Part model, mm, in its own coordinate system. A direction names the side the tool comes from. Round coordinates to 2 decimals unless told otherwise and drop trailing zeros. Order: outer loops, then holes, each group sorted by start corner. A loop starts at its lowest first (then second) coordinate and runs counter-clockwise, first axis right, second up. Notation, with made-up numbers: (-20.5, 17.5) - (34.5, 17.5) arc R26 cw to (34.5, 51.5) - close; hole circle Ø5 at (87.5, -20). An arc over 180 degrees is marked (long way). Return JSON: item names as keys, results as strings. Group by question number.
Item 1: Drop flat-ended pins along their axis: pin 1 (10 mm diameter, centred on x = -17, z = 13, fed in from +Y); pin 2 (14.5 mm diameter, centred on x = 13, y = -3.5, fed in from +Z); pin 3 (7.5 mm diameter, centred on y = -1.5, z = 18, fed in from -X); pin 4 (1 mm diameter, centred on x = 2.5, y = 1, fed in from -Z). Give the stop position or say it passes through.
Item 2: Two-plate mould, pull along X, no slides. Class faces 1 (the face through (-14, 4.826, 20)), 2 (the face through (-0.252, 21.445, 7.776)), 3 (the face through (8, 0, 15.773)): released by +X, released by -X, zero draft, split by the parting line, or undercut.
Item 3: Probe probe 1 along X at (y, z) = (-4.5, 9.5); probe 2 along X at (y, z) = (4, 8); probe 3 along Z at (x, y) = (20, -17). List the from-to ranges inside material, lowest first.
Item 4: Saw through at A-A on z = 26. List the corners of the cut face in (x, y) (1 decimal), and give its area (3 significant figures).
Item 5: Saw through at D-D on x = 4.5. List the corners of the cut face in (y, z).
Item 6: Saw through at B-B on z = 4. State how many separate pieces and enclosed holes the cut face has, and give its area (3 significant figures).
Item 7: Tool access for faces 4 (the face through (43.39, -0.39, 7.78)), 5 (the face through (-14, -4.826, 20)): list every direction of +Z, -Z, +X, -X, +Y, -Y with a clear straight run to the whole face (end or side of a thin tool).
```python
from build123d import *

# Parameters (mm, degrees)
F1_DEPTH = 40.2336
F0_R     = 10.16
F2_DEPTH = 15.7734
F3_R     = 3.302


with BuildPart() as f1:
    # F0 (on Top) → F1 (new body)
    with BuildSketch(Plane.XY):
        with BuildLine():
            ThreePointArc((-27.377507, -23.993331), (-11.81204, -16.223986), (-5.532807, 0))
            ThreePointArc((-5.532807, 0), (-11.81204, 16.223986), (-27.377507, 23.993331))
            ThreePointArc((-27.377507, 23.993331), (-53.730808, 0), (-27.377507, -23.993331))
        make_face()
        with BuildLine():
            ThreePointArc((-16.184043, -4.826), (-43.919307, 0), (-16.184043, 4.826))
            Line((-16.184043, 4.826), (-11.102507, 4.826))
            Line((-11.102507, 4.826), (-11.102507, -4.826))
            Line((-11.102507, -4.826), (-16.184043, -4.826))
        make_face(mode=Mode.SUBTRACT)
    extrude(amount=F1_DEPTH)

    # F0 (on Top) → F2 (join)
    with BuildSketch(Plane.XY):
        with BuildLine():
            ThreePointArc((-27.377507, 23.993331), (-11.81204, 16.223986), (-5.532807, 0))
            ThreePointArc((-5.532807, 0), (-11.81204, -16.223986), (-27.377507, -23.993331))
            Line((-27.377507, -23.993331), (26.125193, -18.96647))
            ThreePointArc((26.125193, -18.96647), (43.393193, 0), (26.125193, 18.96647))
            Line((26.125193, 18.96647), (-27.377507, 23.993331))
        make_face()
        with Locations((24.343193, 0)):
            Circle(F0_R, mode=Mode.SUBTRACT)
    extrude(amount=F2_DEPTH)

    # F3
    f3_edges = [f1.edges().sort_by_distance(p)[0] for p in [
        (-31.886108, 23.993331, 40.2336),
    ]]
    fillet(f3_edges, radius=F3_R)


solid = f1.part
```
Filled in:
{
 "1": {"pin 1": "stops at y = 23.49", "pin 2": "stops at z = 15.77", "pin 3": "stops at x = -53.73", "pin 4": "stops at z = 0"},
 "2": {"face 1": "undercut", "face 2": "released by +X", "face 3": "zero draft"},
 "3": {"probe 1": "x = -53.31 to -43.19, -11.1 to 15.23, 33.45 to 42.85", "probe 2": "x = -53.4 to -43.35, -11.1 to 15, 33.68 to 42.97", "probe 3": "z = 0 to 15.77"},
 "4": {"outline": "(-27.4, -24) arc R24.1 ccw to (-5.5, 0) arc R24.1 ccw to (-27.4, 24) arc R24.1 ccw (long way) to start; hole (-16.2, -4.8) - (-11.1, -4.8) - (-11.1, 4.8) - (-16.2, 4.8) arc R14.3 ccw (long way) to start", "area": "1,140 mm^2"},
 "5": {"outline": "(-21, 0) - (21, 0) - (21, 15.77) - (-21, 15.77) - close"},
 "6": {"separate pieces": "1", "enclosed holes": "2", "area": "2,810 mm^2"},
 "7": {"face 4": "+Z, -Z, +X", "face 5": "+Z, -Z"}
}
